The listing builds one solid part. Answer for the finished solid, in the listing's coordinates (mm). Face numbers are marked on the shaded views. A direction names the side the tool comes from. Round coordinates to 2 decimals unless told otherwise and drop trailing zeros. Write each loop counter-clockwise with the first axis right and the second up, starting at its lowest first coordinate (ties: lowest second). Pieces come first, ordered by that corner, then holes. Notation, with made-up numbers: M 6.25,-11 L 26.25,-11 A12 cw 26.25,1 Z; hole C -17.75,51.5 d9. An arc over 180 degrees is marked long. Put each result on its own line as item: value. Start each with the question number.
```python
from build123d import *

# Parameters (mm, degrees)
SKETCH_1_W          = 14
SKETCH_1_H          = 12
EXTRUDE_1_DEPTH     = 9
FILLET_2_R          = 1
FILLET_3_R          = 1
SKETCH_6_R          = 2.5
EXTRUDE_2_DEPTH     = 11
FILLET_4_R          = 0.5
SKETCH_7_R          = 2
CUT_EXTRUDE_1_DEPTH = 0.5
FILLET_5_R          = 0.5
SKETCH_8_W          = 10
SKETCH_8_H          = 5.607572988
CUT_EXTRUDE_2_DEPTH = 10
SKETCH_9_W          = 10
SKETCH_9_H          = 6
EXTRUDE_3_DEPTH     = 10.1
SKETCH_10_R         = 1.75
CUT_EXTRUDE_3_DEPTH = 0.5
CUT_EXTRUDE_4_DEPTH = 28.828223084
SKETCH_12_W         = 4
SKETCH_12_H         = 5
CUT_EXTRUDE_5_DEPTH = 5


# Some blends are built 0.0001 mm under size
with BuildPart() as part:
    # 草图1 → 凸台-拉伸1 (new body)
    with BuildSketch(Plane(origin=(0, 0, 0), x_dir=(1, 0, 0), z_dir=(0, 1, 0))):
        with Locations((7, 6)):
            Rectangle(SKETCH_1_W, SKETCH_1_H)
    extrude(amount=EXTRUDE_1_DEPTH)

    # 圆角2
    fillet_2_edges = [part.edges().sort_by_distance(p)[0] for p in [
        (14, 9, -6),
        (7, 9, -12),
        (0, 9, -6),
        (7, 9, 0),
    ]]
    fillet(fillet_2_edges, radius=FILLET_2_R)

    # 草图4 → 放样1 section 0
    with BuildSketch(Plane.XZ):
        with BuildLine():
            Line((0, 0), (14, 0))
            Line((14, 0), (14, -12))
            Line((14, -12), (0, -12))
            Line((0, -12), (0, 0))
        make_face()
    # 草图5 → 放样1 section 1
    with BuildSketch(Plane(origin=(0, -11, 0), x_dir=(-1, 0, 0), z_dir=(0, -1, 0))):
        with BuildLine():
            Line((-2, 1), (-12, 1))
            Line((-12, 1), (-12, 11))
            Line((-12, 11), (-2, 11))
            Line((-2, 11), (-2, 1))
        make_face()
    loft()

    # 圆角3
    # the kernel refuses this fillet: 1 mm, written as the material it takes off along each edge
    with BuildSketch(Plane(origin=(14.438278825, 2.410533539, -12.219139413), x_dir=(0.015936381457793344, 0.08765009801785527, 0.9960238411119947), z_dir=(-0.1781741612749496, -0.9799578870122228, 0.0890870806374748)), Plane(origin=(14.438278825, 2.410533539, 0.219139413), x_dir=(-0.9839989676081822, 0.17744243678180333, 0.016131130616527562), z_dir=(-0.1781741612749496, -0.9799578870122228, -0.08908708063747467))) as fillet_3_piece_1:
        with BuildLine():
            CenterArc((FILLET_3_R * 0.983933522321, FILLET_3_R), FILLET_3_R, 180.927975892, 89.072024108)
            Line((-FILLET_3_R * 0.0159353215369, FILLET_3_R * 0.983804473396), (0, 0))
            Line((0, 0), (FILLET_3_R * 0.983933522321, 0))
        make_face()
    extrude(amount=16.144639772, mode=Mode.SUBTRACT)
    with BuildSketch(Plane(origin=(-0.438278825, 2.410533539, -12.219139413), x_dir=(-0.015936381457791863, 0.08765009801785537, 0.9960238411119947), z_dir=(0.1781741612749496, -0.9799578870122228, 0.08908708063747463)), Plane(origin=(-0.438278825, 2.410533539, 0.219139413), x_dir=(0.9839989676081822, 0.17744243678180333, 0.016131130616527607), z_dir=(0.1781741612749496, -0.9799578870122228, -0.0890870806374748))) as fillet_3_piece_2:
        with BuildLine():
            CenterArc((FILLET_3_R * 0.983933522321, -FILLET_3_R), FILLET_3_R, 90, 89.072024108)
            Line((-FILLET_3_R * 0.0159353215369, -FILLET_3_R * 0.983804473396), (0, 0))
            Line((0, 0), (FILLET_3_R * 0.983933522321, 0))
        make_face()
    extrude(amount=16.144639772, mode=Mode.SUBTRACT)

    # 草图6 → 凸台-拉伸2 (add)
    with BuildSketch(Plane.XZ.offset(11)):
        with Locations(Location((7, -6, 0), (0, 0, 270))):
            Circle(SKETCH_6_R)
    extrude(amount=EXTRUDE_2_DEPTH)

    # 圆角4
    fillet_4_edges = [part.edges().sort_by_distance(p)[0] for p in [
        (7, -22, -3.5),
    ]]
    fillet(fillet_4_edges, radius=FILLET_4_R)

    # 草图7 → 切除-拉伸1 (cut)
    with BuildSketch(Plane.XZ.offset(22)):
        with Locations(Location((7, -6, 0), (0, 0, 270))):
            Circle(SKETCH_7_R)
    extrude(amount=-CUT_EXTRUDE_1_DEPTH, mode=Mode.SUBTRACT)

    # 圆角5
    fillet_5_edges = [part.edges().sort_by_distance(p)[0] for p in [
        (7, -21.5, -4),
    ]]
    fillet(fillet_5_edges, radius=FILLET_5_R - 0.0001)  # a hair under: the kernel refuses the full size

    # 草图8 → 切除-拉伸2 (cut)
    with BuildSketch(Plane(origin=(0, 0, -12), x_dir=(-1, 0, 0), z_dir=(0, 0, -1))):
        with Locations((-7, 10.303786494)):
            Rectangle(SKETCH_8_W, SKETCH_8_H)
    extrude(amount=-CUT_EXTRUDE_2_DEPTH, mode=Mode.SUBTRACT)

    # 草图9 → 凸台-拉伸3 (add)
    with BuildSketch(Plane(origin=(0, 0, -2), x_dir=(-1, 0, 0), z_dir=(0, 0, -1))):
        with Locations((-7, 10.5)):
            Rectangle(SKETCH_9_W, SKETCH_9_H)
    extrude(amount=EXTRUDE_3_DEPTH)

    # 草图10 → 切除-拉伸3 (cut)
    with BuildSketch(Plane(origin=(0, 0, -12.1), x_dir=(-1, 0, 0), z_dir=(0, 0, -1))):
        with Locations((-4.5, 10)):
            Circle(SKETCH_10_R)
        with Locations((-9.5, 10)):
            Circle(SKETCH_10_R)
    extrude(amount=-CUT_EXTRUDE_3_DEPTH, mode=Mode.SUBTRACT)

    # 草图11 → 切除-拉伸4 (cut, through all)
    with BuildSketch(Plane.ZY.offset(-2)):
        Polygon((-12.1, 12.5), (-12.1, 13.5), (-9.1, 13.5), align=None)
    extrude(amount=-CUT_EXTRUDE_4_DEPTH, mode=Mode.SUBTRACT)

    # 草图12 → 切除-拉伸5 (cut)
    with BuildSketch(Plane(origin=(0, 13.5, 0), x_dir=(1, 0, 0), z_dir=(0, 1, 0))):
        with Locations((4.5, 5.1)):
            Rectangle(SKETCH_12_W, SKETCH_12_H)
        with Locations((9.5, 5.1)):
            Rectangle(SKETCH_12_W, SKETCH_12_H)
    extrude(amount=-CUT_EXTRUDE_5_DEPTH, mode=Mode.SUBTRACT)


solid = part.part
```
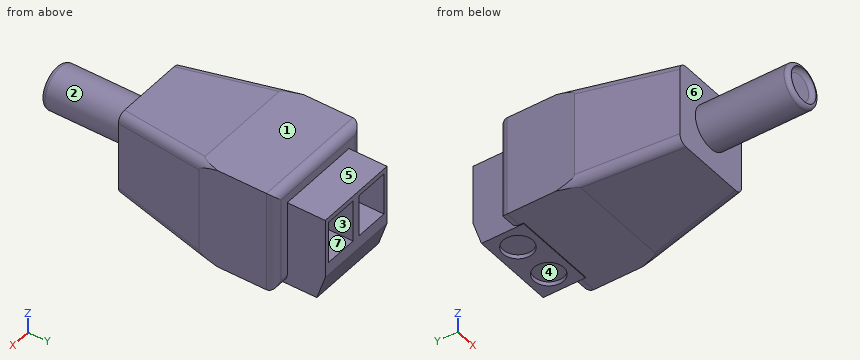
Item 1: Consider line 1 along Y through (x, z) = (11.75, -8); line 2 along Z through (x, y) = (8, 9.5); line 3 along Y through (x, z) = (6.25, -5). Determine where each line is inside the solid, lowest interval first. Write a range as [from, to].
Item 2: Which of the six approach directions +Z, -Z, +X, -X, +Y, -Y give full straight-line access (tool end or side, diameter ignored) to the marked faces 4, 5, 6 and 7?
Item 3: Flat-ended cylindrical pins translate along their axes: pin 1 (5.5 mm diameter, centred on y = 12, z = -5, fed in from +X); pin 2 (2 mm diameter, centred on x = 5.5, y = 11, fed in from +Z); pin 3 (1 mm diameter, centred on x = 4, y = 10, fed in from -Z). Find the tip coordinate at first contact, or state that the pin passes through.
Item 4: Section B-B (y = -16) is taken. Give the vertices of the cut face in (x, z), and give its area (3 significant figures).
Item 5: Section A-A (y = 10) is taken. Give the vertices of the cut face in (x, z), and give its area (3 significant figures).
Item 6: Determine the mould class of the marked faces 1, 2 and 3 for opening direction X: released by +X, released by -X, zero draft, split by the parting line, or undercut.
Output values:
1. line 1: y = [-11, 13.5]
1. line 2: z = [-11.6, -7.6], [-2.6, -2]
1. line 3: y = [-21.5, 8.5]
2. face 4: -Z
2. face 5: +Z, +X, -X, +Y
2. face 6: -Y
2. face 7: +Y
3. pin 1: stops at x = 12
3. pin 2: stops at z = -2
3. pin 3: stops at z = -11.6
4. outline: C 7,-6 d5
4. area: 19.6 mm^2
5. outline: M 2,-12.1 L 2.75,-12.1 L 2.75,-11.6 L 6.25,-11.6 L 6.25,-12.1 L 7.75,-12.1 L 7.75,-11.6 L 11.25,-11.6 L 11.25,-12.1 L 12,-12.1 L 12,-2 L 2,-2 Z; hole M 2.5,-7.6 L 6.5,-7.6 L 6.5,-2.6 L 2.5,-2.6 Z; hole M 7.5,-7.6 L 11.5,-7.6 L 11.5,-2.6 L 7.5,-2.6 Z
5. area: 57.5 mm^2
6. face 1: zero draft
6. face 2: split by the parting line
6. face 3: undercut
